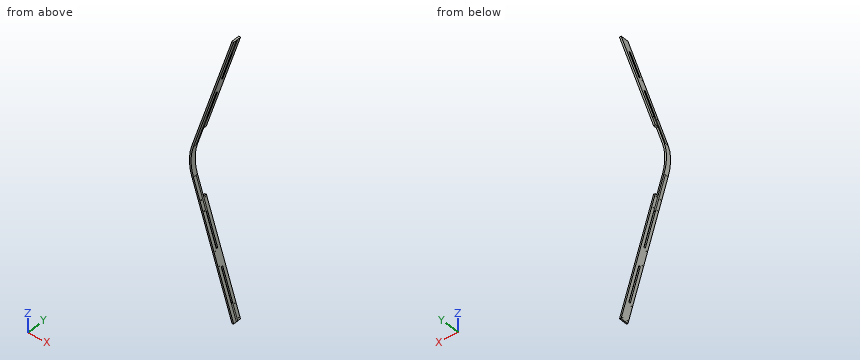
from build123d import *

# Parameters (mm, degrees)
BOSS_EXTRUDE1_DEPTH   = 5
BOSS_EXTRUDE1_2_DEPTH = 5
BOSS_EXTRUDE1_3_DEPTH = 5
BOSS_EXTRUDE1_4_DEPTH = 5
BOSS_EXTRUDE1_5_DEPTH = 5
BOSS_EXTRUDE2_DEPTH   = 20
BOSS_EXTRUDE3_DEPTH   = 20
SKETCH8_R             = 1.5
CUT_EXTRUDE2_DEPTH    = 535.790809635


with BuildPart() as part:
    # Sketch3 → Boss-Extrude1 (new body, symmetric)
    with BuildSketch(Plane(origin=(0, 0, 0), x_dir=(1, 0, 0), z_dir=(0, 1, 0))):
        Polygon((-49.523523643, -856.532206403), (-40.006093165, -853.463246139), (-70.69569581, -758.288941363), (-80.213126288, -761.357901628), align=None)
    extrude(amount=BOSS_EXTRUDE1_DEPTH, both=True)



with BuildPart() as body_2:
    # Sketch3 → Boss-Extrude1 2 (new body, symmetric)
    with BuildSketch(Plane(origin=(0, 0, 0), x_dir=(1, 0, 0), z_dir=(0, 1, 0))):
        with BuildLine():
            Line((-233.661139514, -285.486377751), (-295.040344804, -95.1377682))
            ThreePointArc((-295.040344804, -95.1377682), (-310, 0), (-295.040344804, 95.1377682))
            Line((-295.040344804, 95.1377682), (-233.661139514, 285.486377751))
            Line((-233.661139514, 285.486377751), (-224.143709036, 282.417417486))
            Line((-224.143709036, 282.417417486), (-285.522914326, 92.068807935))
            ThreePointArc((-285.522914326, 92.068807935), (-300, 0), (-285.522914326, -92.068807935))
            Line((-285.522914326, -92.068807935), (-224.143709036, -282.417417486))
            Line((-224.143709036, -282.417417486), (-233.661139514, -285.486377751))
        make_face()
    extrude(amount=BOSS_EXTRUDE1_2_DEPTH, both=True)


with BuildPart() as body_3:
    # Sketch3 → Boss-Extrude1 3 (new body, symmetric)
    with BuildSketch(Plane(origin=(0, 0, 0), x_dir=(1, 0, 0), z_dir=(0, 1, 0))):
        Polygon((-132.074901101, -567.940331812), (-141.592331578, -571.009292077), (-172.281934223, -475.834987302), (-162.764503746, -472.766027037), align=None)
    extrude(amount=BOSS_EXTRUDE1_3_DEPTH, both=True)


with BuildPart() as body_4:
    # Sketch3 → Boss-Extrude1 4 (new body, symmetric)
    with BuildSketch(Plane(origin=(0, 0, 0), x_dir=(1, 0, 0), z_dir=(0, 1, 0))):
        Polygon((-70.69569581, 758.288941363), (-40.006093165, 853.463246139), (-49.523523643, 856.532206403), (-80.213126288, 761.357901628), align=None)
    extrude(amount=BOSS_EXTRUDE1_4_DEPTH, both=True)


with BuildPart() as body_5:
    # Sketch3 → Boss-Extrude1 5 (new body, symmetric)
    with BuildSketch(Plane(origin=(0, 0, 0), x_dir=(1, 0, 0), z_dir=(0, 1, 0))):
        Polygon((-162.764503746, 472.766027037), (-132.074901101, 567.940331812), (-141.592331578, 571.009292077), (-172.281934223, 475.834987302), align=None)
    extrude(amount=BOSS_EXTRUDE1_5_DEPTH, both=True)


with BuildPart() as part_1:
    add(part.part)

    add(body_2.part)  # Boss-Extrude2 merges body 2

    add(body_3.part)  # Boss-Extrude2 merges body 3

    add(body_4.part)  # Boss-Extrude2 merges body 4

    add(body_5.part)  # Boss-Extrude2 merges body 5
    # Sketch4 → Boss-Extrude2 (add)
    with BuildSketch(Plane(origin=(0, 5, 0), x_dir=(1, 0, 0), z_dir=(0, 1, 0))):
        Polygon((-49.523523643, -856.532206403), (-258.21282163, -209.34693393), (-248.695391152, -206.277973666), (-40.006093165, -853.463246139), align=None)
        Polygon((-49.523523643, 856.532206403), (-40.006093165, 853.463246139), (-248.695391152, 206.277973666), (-258.21282163, 209.34693393), align=None)
    extrude(amount=BOSS_EXTRUDE2_DEPTH)

    # Sketch5 → Boss-Extrude3 (add)
    with BuildSketch(Plane.XZ.offset(5)):
        with BuildLine():
            Line((-49.523523643, 856.532206403), (-40.006093165, 853.463246139))
            Line((-40.006093165, 853.463246139), (-285.522914326, 92.068807935))
            ThreePointArc((-285.522914326, 92.068807935), (-300, 0), (-285.522914326, -92.068807935))
            Line((-285.522914326, -92.068807935), (-40.006093165, -853.463246139))
            Line((-40.006093165, -853.463246139), (-49.523523643, -856.532206403))
            Line((-49.523523643, -856.532206403), (-295.040344804, -95.1377682))
            ThreePointArc((-295.040344804, -95.1377682), (-310, 0), (-295.040344804, 95.1377682))
            Line((-295.040344804, 95.1377682), (-49.523523643, 856.532206403))
        make_face()
    extrude(amount=BOSS_EXTRUDE3_DEPTH)

    # Sketch8 → Cut-Extrude2 (cut, through all)
    with BuildSketch(Plane(origin=(-295.040344804, 0, 95.1377682), x_dir=(0.306896026, 0, 0.951743048), z_dir=(-0.951743048, 0, 0.306896026))):
        with Locations((790, 15)):
            Circle(SKETCH8_R)
        with Locations((710, 15)):
            Circle(SKETCH8_R)
        with Locations((410, 15)):
            Circle(SKETCH8_R)
        with Locations((490, 15)):
            Circle(SKETCH8_R)
        with Locations((130, 15)):
            Circle(SKETCH8_R)
        with Locations((190, 15)):
            Circle(SKETCH8_R)
        with Locations((790, -15)):
            Circle(SKETCH8_R)
        with Locations((190, -15)):
            Circle(SKETCH8_R)
        with Locations((130, -15)):
            Circle(SKETCH8_R)
        with Locations((490, -15)):
            Circle(SKETCH8_R)
        with Locations((410, -15)):
            Circle(SKETCH8_R)
        with Locations((710, -15)):
            Circle(SKETCH8_R)
    cut_extrude2 = extrude(amount=-CUT_EXTRUDE2_DEPTH, mode=Mode.SUBTRACT)

    # Mirror1: Cut-Extrude2 across plane
    add(cut_extrude2.mirror(Plane.XY), mode=Mode.SUBTRACT)


solid = part_1.part
Input: part model. Units: mm. Frame: model coordinates. Coordinates: 2 decimals unless noted, no trailing zeros. Order: outer loops, then holes, each group sorted by start corner. A loop starts at its lowest first (then second) coordinate and runs counter-clockwise, first axis right, second up.
1. Cut plane B-B, the plane z = 352.5. Return loops of the section in (x, y), plus the area to 3 significant figures.
Checked values:
outline: (-212.05, -25) - (-201.55, -25) - (-201.55, -5) - (-212.05, -5) - close; (-212.05, 5) - (-201.55, 5) - (-201.55, 25) - (-212.05, 25) - close
area: 420 mm2
2. Cut plane A-A, the plane x = -207. Return loops of the section in (y, z).
Checked values:
outline: (-25, -368.17) - (-5, -368.17) - (-5, -335.58) - (-25, -335.58) - close; (-25, 335.58) - (-5, 335.58) - (-5, 368.17) - (-25, 368.17) - close; (5, -368.17) - (25, -368.17) - (25, -335.58) - (5, -335.58) - close; (5, 335.58) - (25, 335.58) - (25, 368.17) - (5, 368.17) - close
3. Ray query, line 1 along X through (y, z) = (-5, -556.5); line 2 along X through (y, z) = (-10.5, 562). Return the intervals inside material, ascending.
Checked values:
line 1: x = -146.27 to -135.76
line 2: x = -144.5 to -133.99
4. Contact query for flat-ended pins moving along their axis: P1, Ø21.5, axis at x = -215.5, z = -399, coming from the -Y side; P2, Ø3, axis at y = -19.5, z = 654, coming from the -X side; P3, Ø6, axis at y = 18.5, z = 302, coming from the -X side; P4, Ø8, axis at y = -5.5, z = 153, coming from the -X side. Output: stop coordinate, or through.
Checked values:
P1: passes through
P2: stops at x = -115.32
P3: stops at x = -229.3
P4: stops at x = -277.67
